Study the drawing (mm; zero at the part's minimum x, y, z) and answer. A direction names the side the tool comes from. Coordinates: 2 decimals unless noted, no trailing zeros. Write each loop counter-clockwise with the first axis right and the second up, starting at its lowest first coordinate (ties: lowest second). Pieces come first, ordered by that corner, then holes. Notation, with made-up numbers: (-6, -11.75) -> (40, -11.75) arc R28 ccw to (40, 27.25) -> close; hole circle Ø2 at (13.25, -39). An arc over 180 degrees is marked (long way). Answer in a Markdown table with one row per item. Add a question column.
Item 1: For a pull along Z with two mould halves and no side action, classify the marked faces 3, 4, 5 and 6 as +Z half, -Z half, draft (parallel to the pull), parting line (faces both ways), or undercut.
Item 2: Section C-C on y = 23 is taken. Write down the section's boundary in (x, z), then the cut area to 3 significant figures.
Item 3: Given pin 1 Ø5 at (x, z) = (79, 18.5) entering from -Y; pin 2 Ø5 at (x, z) = (80, 20) entering from +Y, each flat-ended and moving along its own axis, determine where each tip first touches the part or whether it passes through.
Item 4: Section B-B on z = 20 is taken. Write down the section's boundary in (x, y) (3 decimals), then the cut area to 3 significant figures.
Item 5: Straight lines are drawn through the part: line 1 (Z direction, x = 10, y = 25.5); line 2 (Z direction, x = 65, y = 4.75); line 3 (X direction, y = 2, z = 27.5) (1 decimal). For each, find the intervals that lie inside material, in ascending order. Write a range as from..to.
Item 6: Which of the six approach directions +Z, -Z, +X, -X, +Y, -Y give full straight-line access (tool end or side, diameter ignored) to the marked faces 1 and 2?
Item 7: Section D-D on y = 3 is taken. Write down the section's boundary in (x, z) (3 decimals).
Item 8: Section A-A on x = 10 is taken. Write down the section's boundary in (y, z) (3 decimals), then the cut area to 3 significant figures.
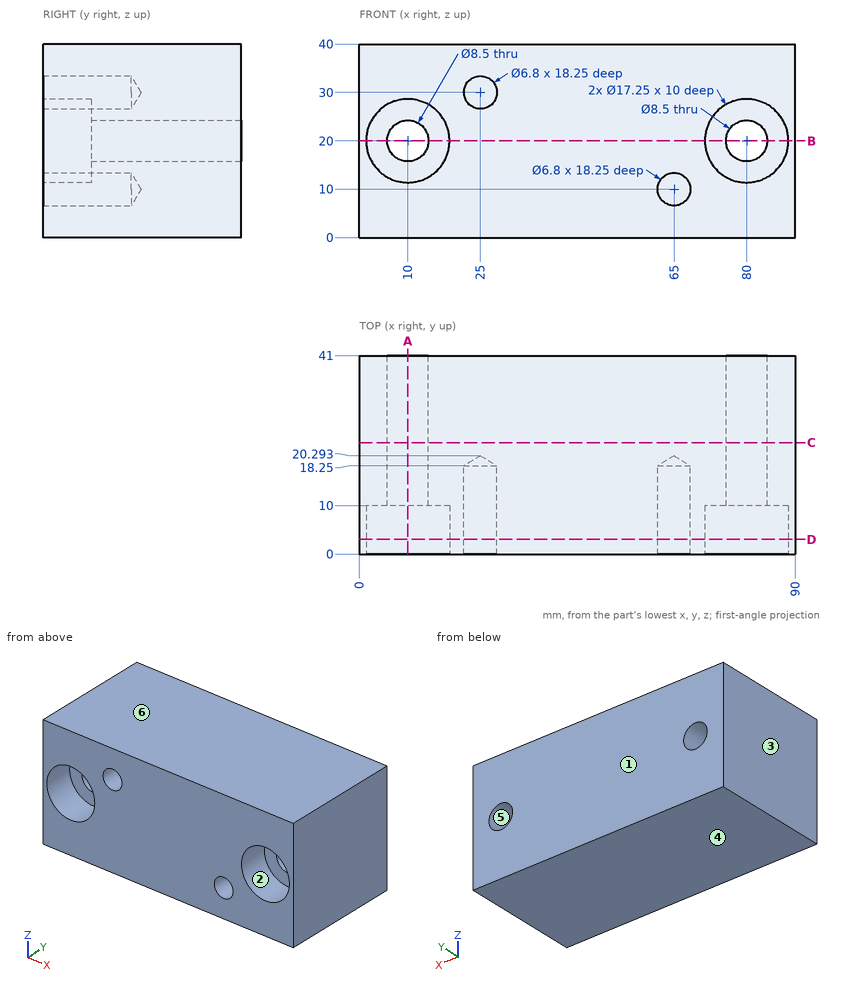
Results below:
| question | item | result |
|---|---|---|
| 1 | face 3 | draft |
| 1 | face 4 | -Z half |
| 1 | face 5 | undercut |
| 1 | face 6 | +Z half |
| 2 | outline | (0, 0) -> (90, 0) -> (90, 40) -> (0, 40) -> close; hole circle Ø8.5 at (10, 20); hole circle Ø8.5 at (80, 20) |
| 2 | area | 3,490 mm2 |
| 3 | pin 1 | stops at y = 10 |
| 3 | pin 2 | passes through |
| 4 | outline | (0, 0) -> (1.375, 0) -> (1.375, 10) -> (5.75, 10) -> (5.75, 41) -> (0, 41) -> close; (14.25, 10) -> (18.625, 10) -> (18.625, 0) -> (71.375, 0) -> (71.375, 10) -> (75.75, 10) -> (75.75, 41) -> (14.25, 41) -> close; (84.25, 10) -> (88.625, 10) -> (88.625, 0) -> (90, 0) -> (90, 41) -> (84.25, 41) -> close |
| 4 | area | 2,820 mm2 |
| 5 | line 1 | z = 0..15.75, 24.25..40 |
| 5 | line 2 | z = 0..6.6, 13.4..40 |
| 5 | line 3 | x = 0..5.7, 14.3..22.7, 27.3..75.7, 84.3..90 |
| 6 | face 1 | +Z, -Z, +X, -X, +Y |
| 6 | face 2 | -Y |
| 7 | outline | (0, 0) -> (90, 0) -> (90, 40) -> (0, 40) -> close; hole circle Ø17.25 at (10, 20); hole circle Ø6.8 at (25, 30); hole circle Ø6.8 at (65, 10); hole circle Ø17.25 at (80, 20) |
| 8 | outline | (0, 0) -> (41, 0) -> (41, 15.75) -> (10, 15.75) -> (10, 11.375) -> (0, 11.375) -> close; (0, 28.625) -> (10, 28.625) -> (10, 24.25) -> (41, 24.25) -> (41, 40) -> (0, 40) -> close |
| 8 | area | 1,200 mm2 |
